Geometry check sheet. Reference: drawing and pictorial views, mm from the part's lowest x, y, z. Round coordinates to 2 decimals unless told otherwise and drop trailing zeros. Write each loop counter-clockwise with the first axis right and the second up, starting at its lowest first coordinate (ties: lowest second). Pieces come first, ordered by that corner, then holes.
Item 1: Material ranges on line 1 along Y through (x, z) = (25.5, 24.5); line 2 along X through (y, z) = (88, 31.5); line 3 along Z through (x, y) = (91.5, 116.5), recorded low to high.
Item 2: Section check D-D, the plane x = 24. Record the cut outline in (y, z).
Item 3: Section check C-C, the plane y = 138. Record the cut outline in (x, z).
Item 4: Section check A-A, the plane x = 48. Record the cut outline in (y, z), plus the area to 3 significant figures.
Item 5: Section check B-B, the plane z = 29.5. Record the cut outline in (x, y).
Item 6: Release check for a two-part mould opening along Y. For the marked faces 1, 2, 3 and 4 record: pulls with the +Y half, pulls with the -Y half, needs draft (parallel to the pull), parting line crosses it, or undercut.
Item 7: Depth check by flat-ended pin: pin 1 (16 mm diameter, centred on y = 46, z = 12.5, fed in from -X); pin 2 (1.5 mm diameter, centred on x = 49.5, y = 87, fed in from +Z); pin 3 (4 mm diameter, centred on x = 83.5, y = 35.5, fed in from -Z); pin 4 (2 mm diameter, centred on y = 22, z = 4, fed in from +X). Enter the tip coordinate at first touch or a pass-through.
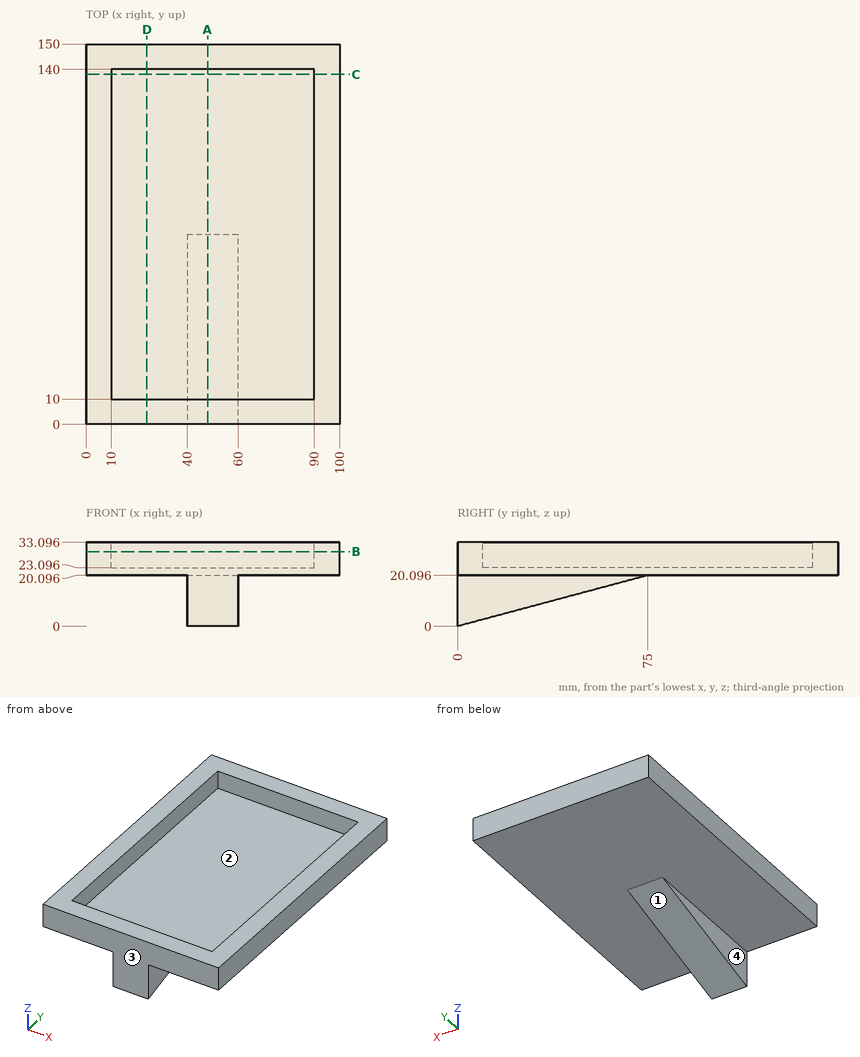
Values found:
1. line 1: y = 0 to 10, 140 to 150
1. line 2: x = 0 to 10, 90 to 100
1. line 3: z = 20.1 to 33.1
2. outline: (0, 20.1) - (150, 20.1) - (150, 33.1) - (140, 33.1) - (140, 23.1) - (10, 23.1) - (10, 33.1) - (0, 33.1) - close
3. outline: (0, 20.1) - (100, 20.1) - (100, 33.1) - (90, 33.1) - (90, 23.1) - (10, 23.1) - (10, 33.1) - (0, 33.1) - close
4. outline: (0, 0) - (75, 20.1) - (150, 20.1) - (150, 33.1) - (140, 33.1) - (140, 23.1) - (10, 23.1) - (10, 33.1) - (0, 33.1) - close
4. area: 1,400 mm2
5. outline: (0, 0) - (100, 0) - (100, 150) - (0, 150) - close; hole (10, 10) - (90, 10) - (90, 140) - (10, 140) - close
6. face 1: pulls with the +Y half
6. face 2: undercut
6. face 3: pulls with the -Y half
6. face 4: needs draft
7. pin 1: stops at x = 0
7. pin 2: stops at z = 23.1
7. pin 3: stops at z = 20.1
7. pin 4: passes through
